Can you work these out from the drawing? Everything is in mm from the part's minimum corner. Round coordinates to 2 decimals unless told otherwise and drop trailing zeros. Write each loop counter-clockwise with the first axis right and the second up, starting at its lowest first coordinate (ties: lowest second). Pieces come first, ordered by that corner, then holes. Notation, with made-up numbers: (1.5, 46.5) - (38.5, 46.5) arc R31 cw to (38.5, 77.5) - close; hole circle Ø11 at (67, -10.75). An arc over 180 degrees is marked (long way). One line per item, written item: value. Start each with the question number.
(1) If I drill on L1, parallel to Z at x = 25.4, y = 2.1; L2, parallel to Z at x = 26.5, y = 3.85; L3, parallel to X at y = 1.05, z = 13.5, over which ranges is the centre line in solid material (lowest first)? Write a range as from..to.
(2) I want a section at D-D on x = 13.5. List the corners of the cut face in (y, z) for me (1 decimal), plus the area to 3 significant figures.
(3) I'm going to push flat-ended pins straight in: pin 1 Ø4 at (x, z) = (25.4, 63.5) entering from +Y; pin 2 Ø1.5 at (y, z) = (3, 33) entering from +X. Where does each tip first touch, or does it pass through?
(4) I want a section at C-C on z = 38.1. List the corners of the cut face in (x, y) for me (1 decimal), plus the area to 3 significant figures.
(5) I want a section at A-A on z = 12.7. List the corners of the cut face in (x, y) for me (1 decimal), plus the area to 3 significant figures.
(6) I want a section at B-B on y = 3.7. List the corners of the cut face in (x, z) for me, plus the area to 3 significant figures.
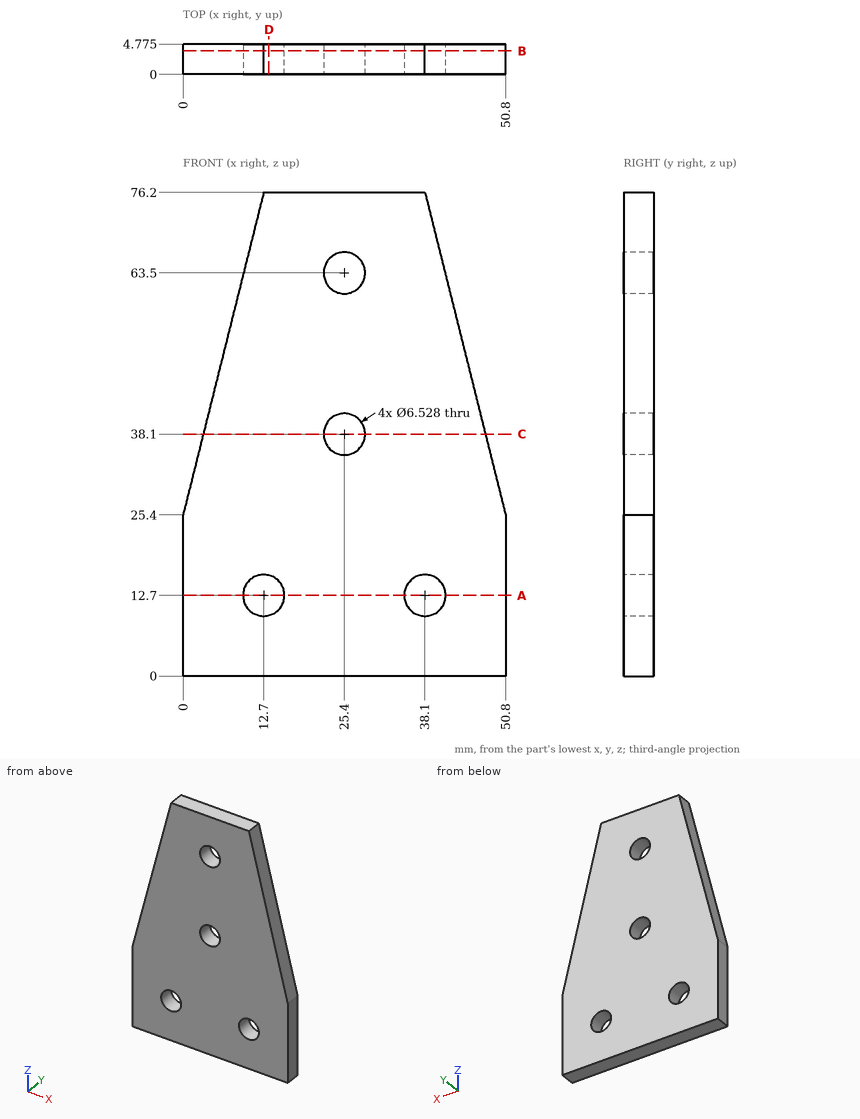
Established:
1. L1: 0..34.84, 41.36..60.24, 66.76..76.2
1. L2: 0..35.03, 41.17..60.43, 66.57..76.2
1. L3: 0..9.54, 15.86..34.94, 41.26..50.8
2. outline: (0, 0) - (4.8, 0) - (4.8, 9.5) - (0, 9.5) - close; (0, 15.9) - (4.8, 15.9) - (4.8, 76.2) - (0, 76.2) - close
2. area: 334 mm2
3. pin 1: through
3. pin 2: x = 49.09
4. outline: (3.2, 0) - (22.1, 0) - (22.1, 4.8) - (3.2, 4.8) - close; (28.7, 0) - (47.6, 0) - (47.6, 4.8) - (28.7, 4.8) - close
4. area: 181 mm2
5. outline: (0, 0) - (9.4, 0) - (9.4, 4.8) - (0, 4.8) - close; (16, 0) - (34.8, 0) - (34.8, 4.8) - (16, 4.8) - close; (41.4, 0) - (50.8, 0) - (50.8, 4.8) - (41.4, 4.8) - close
5. area: 180 mm2
6. outline: (0, 0) - (50.8, 0) - (50.8, 25.4) - (38.1, 76.2) - (12.7, 76.2) - (0, 25.4) - close; hole circle Ø6.53 at (12.7, 12.7); hole circle Ø6.53 at (25.4, 38.1); hole circle Ø6.53 at (25.4, 63.5); hole circle Ø6.53 at (38.1, 12.7)
6. area: 3,090 mm2
